Work out the finished part from the listing and answer in its coordinate system (mm). Coordinates: 2 decimals unless noted, no trailing zeros. Loops run counter-clockwise (first coordinate to the right, second up) from the corner with the lowest first, then second, coordinate; pieces in that order, holes last. Notation, with made-up numbers: (30.25, 11) -> (64.25, 11) arc R19 ccw to (64.25, 34) -> close; hole circle Ø4 at (-3, 66.25). An arc over 180 degrees is marked (long way). Use a Markdown table: item, result.
from build123d import *

# Parameters (mm, degrees)
SKETCH1_R           = 30
BOSS_EXTRUDE1_DEPTH = 16
SKETCH4_R           = 2.5
CUT_EXTRUDE2_DEPTH  = 6


with BuildPart() as part:
    # Sketch1 → Boss-Extrude1 (new body)
    with BuildSketch(Plane.XY):
        Circle(SKETCH1_R)
    extrude(amount=BOSS_EXTRUDE1_DEPTH)

    # Sketch3 → Cut-Revolve2 (revolve, cut)
    with BuildSketch(Plane(origin=(0, 0, 0), x_dir=(1, 0, 0), z_dir=(0, 1, 0)), mode=Mode.PRIVATE) as cut_revolve2_sk:
        with BuildLine():
            Line((0, -16), (30, -16))
            ThreePointArc((30, -16), (15.076344301, -13.728961616), (0, -12.969384567))
            Line((0, -12.969384567), (0, -16))
        make_face()
    revolve(cut_revolve2_sk.sketch.rotate(Axis((0, 0, 12.969384567), (0, 0, 1)), 180), axis=Axis((0, 0, 12.969384567), (0, 0, 1)), mode=Mode.SUBTRACT)

    # Sketch4 → Cut-Extrude2 (cut)
    with BuildSketch(Plane(origin=(0, 0, 0), x_dir=(-1, 0, 0), z_dir=(0, 0, -1))):
        with Locations((-16, 0)):
            Circle(SKETCH4_R)
    extrude(amount=-CUT_EXTRUDE2_DEPTH, mode=Mode.SUBTRACT)


solid = part.part
Q1. Consider line 1 (Y direction, x = 16, z = 2.1); line 2 (Y direction, x = 14, z = 5); line 3 (Y direction, x = -16, z = 7.5). Determine where each line is inside the solid, lowest interval first. Write a range as [from, to].
Solved:
| item | result |
|---|---|
| line 1 | [-25.38, -2.5], [2.5, 25.38] |
| line 2 | [-26.53, -1.5], [1.5, 26.53] |
| line 3 | [-25.38, 25.38] |
Q2. Section B-B on x = 16 is taken. Determine the outline of the cut face in (y, z).
Solved:
| item | result |
|---|---|
| outline | (-25.38, 0) -> (-2.5, 0) -> (-2.5, 6) -> (2.5, 6) -> (2.5, 0) -> (25.38, 0) -> (25.38, 16) arc R149.14 cw to (-25.38, 16) -> close |
Q3. Given pin 1 Ø6 at (x, y) = (-14.5, 18) entering from +Z; pin 2 Ø5.5 at (x, y) = (15, -1) entering from -Z; pin 3 Ø5 at (x, y) = (-20.5, 13) entering from +Z; pin 4 Ø8 at (x, z) = (-3.5, 12) entering from +Y, each flat-ended and moving along its own axis, determine where each tip first touches the part or whether it passes through.
Solved:
| item | result |
|---|---|
| pin 1 | z = 15.26 |
| pin 2 | z = 0 |
| pin 3 | z = 15.38 |
| pin 4 | y = 30 |
Q4. Section C-C on z = 2.75 is taken. Determine the outline of the cut face in (x, y), and give its area (3 significant figures).
Solved:
| item | result |
|---|---|
| outline | circle Ø60 at (0, 0); hole circle Ø5 at (16, 0) |
| area | 2,810 mm² |
Q5. Determine the mould class of faces 1 (the cylindrical face through (-29.97, 1.32, 7.89)), 2 (the flat face through (0, 0, 0)), 3 (the flat face through (16, 0, 6)) for opening direction X: pulls with the +X half, pulls with the -X half, needs draft (parallel to the pull), parting line crosses it, or undercut.
Solved:
| item | result |
|---|---|
| face 1 | parting line crosses it |
| face 2 | needs draft |
| face 3 | undercut |
Q6. Section A-A on y = 0 is taken. Determine the outline of the cut face in (x, z), and give its area (3 significant figures).
Solved:
| item | result |
|---|---|
| outline | (-30, 0) -> (13.5, 0) -> (13.5, 6) -> (18.5, 6) -> (18.5, 0) -> (30, 0) -> (30, 16) arc R150 cw to (-30, 16) -> close |
| area | 809 mm² |
Q7. Section D-D on z = 9 is taken. Determine the outline of the cut face in (x, y).
Solved:
| item | result |
|---|---|
| outline | circle Ø60 at (0, 0) |
